```python
from build123d import *

# Parameters (mm, degrees)
EXTRUDE1_DEPTH = 15.407108717
EXTRUDE2_START = 7.422870335
EXTRUDE2_DEPTH = 7.422870335
SKETCH3_R      = 3.81
EXTRUDE3_DEPTH = 37.782065936
SKETCH4_R      = 1.016
EXTRUDE4_DEPTH = 41.456758632
SKETCH6_W      = 2.451904957
SKETCH6_H      = 3.748582847
SKETCH6_W_2    = 11.438391631
EXTRUDE6_DEPTH = 39.80458612


with BuildPart() as part:
    # Sketch1 → Extrude1 (new body)
    with BuildSketch(Plane.XY):
        with BuildLine():
            Line((-7.138522943, 30.753654662), (-7.138522943, 0))
            ThreePointArc((-7.138522943, 0), (0.445823167, -7.124587813), (7.08283683, 0.889905749))
            Line((7.08283683, 0.889905749), (5.932301807, 10.047113518))
            ThreePointArc((5.932301807, 10.047113518), (5.707297096, 10.62465377), (5.235742646, 11.026917691))
            Line((5.235742646, 11.026917691), (-0.692002916, 13.961994048))
            ThreePointArc((-0.692002916, 13.961994048), (-1.163557366, 14.364257969), (-1.388562077, 14.941798222))
            Line((-1.388562077, 14.941798222), (-3.404561048, 30.987308419))
            ThreePointArc((-3.404561048, 30.987308419), (-5.381286902, 32.624287275), (-7.138522943, 30.753654662))
        make_face()
    extrude(amount=EXTRUDE1_DEPTH)

    # Sketch2 → Extrude2 (add)
    with BuildSketch(Plane(origin=(0, 0, 0), x_dir=(-1, 0, 0), z_dir=(0, 0, -1)).offset(EXTRUDE2_START)):
        with BuildLine():
            Line((1.388562077, 14.941798222), (3.404561048, 30.987308419))
            ThreePointArc((3.404561048, 30.987308419), (5.381286902, 32.624287275), (7.138522943, 30.753654662))
            Line((7.138522943, 30.753654662), (7.138522943, 8.467771223))
            ThreePointArc((7.138522943, 8.467771223), (6.680781174, 7.362684837), (5.575694788, 6.904943069))
            Line((5.575694788, 6.904943069), (-5.473496233, 6.904943069))
            ThreePointArc((-5.473496233, 6.904943069), (-6.038205752, 7.159804295), (-6.220680789, 7.751880259))
            Line((-6.220680789, 7.751880259), (-5.932301807, 10.047113518))
            ThreePointArc((-5.932301807, 10.047113518), (-5.707297096, 10.62465377), (-5.235742646, 11.026917691))
            Line((-5.235742646, 11.026917691), (0.692002916, 13.961994048))
            ThreePointArc((0.692002916, 13.961994048), (1.163557366, 14.364257969), (1.388562077, 14.941798222))
        make_face()
    extrude(amount=-EXTRUDE2_DEPTH)

    # Sketch3 → Extrude3 (cut, through all)
    with BuildSketch(Plane(origin=(0, 0, 0), x_dir=(-1, 0, 0), z_dir=(0, 0, -1))):
        Circle(SKETCH3_R)
    extrude(amount=-EXTRUDE3_DEPTH, mode=Mode.SUBTRACT)

    # Sketch4 → Extrude4 (cut, through all)
    with BuildSketch(Plane(origin=(0, 0, -7.422870335), x_dir=(-1, 0, 0), z_dir=(0, 0, -1))):
        with Locations((5.264231519, 30.753654662)):
            Circle(SKETCH4_R)
    extrude(amount=-EXTRUDE4_DEPTH, mode=Mode.SUBTRACT)

    # Sketch6 → Extrude6 (cut, through all)
    with BuildSketch(Plane.ZY.offset(7.138522943)):
        with Locations((-3.656917857, 30.753654662)):
            Rectangle(SKETCH6_W, SKETCH6_H)
        with Locations((7.490088589, 30.753654662)):
            Rectangle(SKETCH6_W_2, SKETCH6_H)
    extrude(amount=-EXTRUDE6_DEPTH, mode=Mode.SUBTRACT)


solid = part.part
```
Work out the finished part from the listing and answer in its coordinate system (mm). A direction names the side the tool comes from. Give positions to 0.01 mm unless a question says otherwise; leave off trailing zeros. Loops run counter-clockwise (first coordinate to the right, second up) from the corner with the lowest first, then second, coordinate; pieces in that order, holes last. Notation, with made-up numbers: (-28, 0.5) -> (24, 0.5) arc R24 cw to (24, 36.5) -> close; hole circle Ø5 at (37, -35.5). An arc over 180 degrees is marked (long way). One line per question, with ' | ' between items. Start each with the question number.
1) Section B-B, the plane x = 0 is taken. Determine the outline of the cut face in (y, z).
2) Section D-D, the plane z = 10.5 is taken. Determine the outline of the cut face in (x, y), then the cut area to 3 significant figures.
3) Determine the mould class of faces 6 (the face through (-4, 30, 13.209)), 7 (the face through (-2, 9, 15.407)), 8 (the face through (0, 4, 0)) for opening direction Z: +Z half, -Z half, draft (parallel to the pull), parting line (faces both ways), or undercut.
4) Section C-C, the plane y = 3 is taken. Determine the outline of the cut face in (x, z).
5) For faces 1 (the face through (-6.69, 7.37, -3.76)), 2 (the face through (-5.342, 32.626, -6.171)), 3 (the face through (0, 6.905, -4)), 4 (the face through (-4, 30, 1.771)), 5 (the face through (-2.382, 22.852, 3.832)), determine the directions among +Z, -Z, +X, -X, +Y, -Y from which every point of the face is accessible in a straight line to the end or side of a thin tool.
6) Straight lines are drawn through the part: L1, parallel to Z at x = -4.25, y = 29; L2, parallel to Y at x = -0.5, z = 13; L3, parallel to X at y = 1, z = 0.5. For each, find the intervals that lie inside material, in ascending order.
7) Each of these flat-tipped pins is pushed along its axis until it touches: pin 1 (3 mm diameter, centred on x = -5, y = 31.5, fed in from +Z); pin 2 (2 mm diameter, centred on x = -1, z = -5.5, fed in from -Y); pin 3 (3 mm diameter, centred on x = -4.5, z = 6, fed in from +Y); pin 4 (1 mm diameter, centred on y = 19, z = -4, fed in from +X). Where does it stop, or does it pass through?
8) Section A-A, the plane z = -1.5 is taken. Determine the outline of the cut face in (x, y).
Resolved:
1) outline: (-7.14, 0) -> (-3.81, 0) -> (-3.81, 15.41) -> (-7.14, 15.41) -> close; (3.81, 0) -> (6.9, 0) -> (6.9, -7.42) -> (13.62, -7.42) -> (13.62, 15.41) -> (3.81, 15.41) -> close
2) outline: (-7.14, 0) arc R7.14 ccw (long way) to (7.08, 0.89) -> (5.93, 10.05) arc R1.27 ccw to (5.24, 11.03) -> (-0.69, 13.96) arc R1.27 cw to (-1.39, 14.94) -> (-3.14, 28.88) -> (-7.14, 28.88) -> close; hole circle Ø7.62 at (0, 0) | area: 286 mm2
3) face 6: undercut | face 7: +Z half | face 8: -Z half
4) outline: (-7.14, 0) -> (-2.35, 0) -> (-2.35, 15.41) -> (-7.14, 15.41) -> close; (2.35, 0) -> (6.82, 0) -> (6.82, 15.41) -> (2.35, 15.41) -> close
5) face 1: -Z, -X, -Y | face 2: +Z, -Z, +Y | face 3: -Z, +X, -X, -Y | face 4: +X, -X, +Y | face 5: +Z, -Z, +X, +Y
6) L1: -7.42 to -4.88, -2.43 to 1.77, 13.21 to 15.41 | L2: -7.12 to -3.78, 3.78 to 13.87 | L3: -7.14 to -3.68, 3.68 to 7.07
7) pin 1: z = 15.41 | pin 2: y = 6.9 | pin 3: y = 28.88 | pin 4: x = -1.84
8) outline: (-7.14, 8.47) arc R1.56 ccw to (-5.58, 6.9) -> (5.47, 6.9) arc R0.75 ccw to (6.22, 7.75) -> (5.93, 10.05) arc R1.27 ccw to (5.24, 11.03) -> (-0.69, 13.96) arc R1.27 cw to (-1.39, 14.94) -> (-3.4, 30.99) arc R1.87 ccw to (-7.14, 30.75) -> close; hole circle Ø2.03 at (-5.26, 30.75)
